For this review, use the dimensioned drawing (mm, ordinates from the lowest corner) and the shaded views. A direction names the side the tool comes from. Round coordinates to 2 decimals unless told otherwise and drop trailing zeros. Write each loop counter-clockwise with the first axis right and the second up, starting at its lowest first coordinate (ties: lowest second). Pieces come first, ordered by that corner, then holes. Notation, with made-up numbers: (1.25, 29.5) - (28.25, 29.5) arc R36 cw to (28.25, 65.5) - close; hole circle Ø5 at (-34.75, 20.25). An arc over 180 degrees is marked (long way). Return JSON: item names as keys, results as strings.
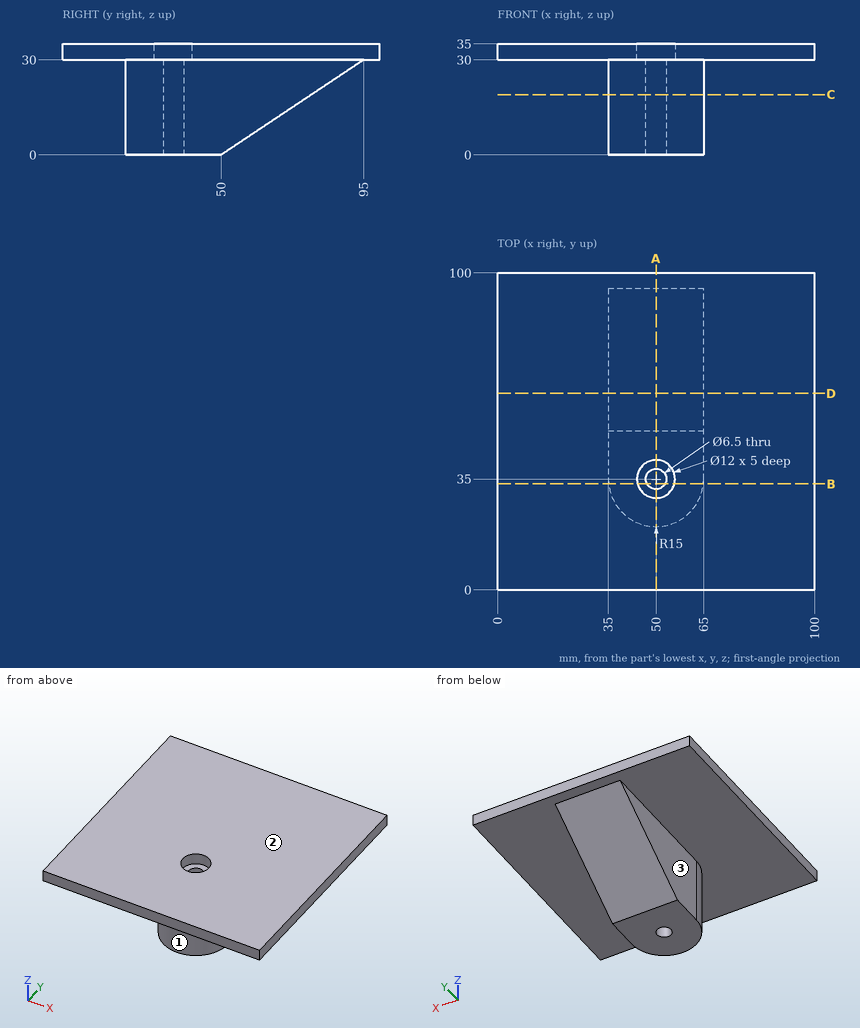
(1) Clearance check with flat-ended pins moving along their axes: pin 1 Ø5 at (x, z) = (34.5, 25.5) entering from -Y; pin 2 Ø5 at (y, z) = (82, 20) entering from +X; pin 3 Ø1 at (y, z) = (70.5, 22.5) entering from -X. State where each tip first meets the part, or that it passes through.
Filled in:
{"pin 1": "stops at y = 27.52", "pin 2": "stops at x = 65", "pin 3": "stops at x = 35"}
(2) Add section A-A (x = 50). Write out the cut boundary in (y, z).
Filled in:
{"outline": "(0, 30) - (20, 30) - (20, 0) - (31.75, 0) - (31.75, 30) - (29, 30) - (29, 35) - (0, 35) - close; (38.25, 0) - (50, 0) - (95, 30) - (100, 30) - (100, 35) - (41, 35) - (41, 30) - (38.25, 30) - close"}
(3) Add section C-C (z = 19). Write out the cut boundary in (x, y), plus the area to 3 significant figures.
Filled in:
{"outline": "(35, 35) arc R15 ccw to (65, 35) - (65, 78.5) - (35, 78.5) - close; hole circle Ø6.5 at (50, 35)", "area": "1,630 mm2"}
(4) Wall thickness on line 1 (Y direction, x = 50, z = 31.2); line 2 (X direction, y = 39.5, z = 9.5); line 3 (Z direction, x = 27, y = 89): over which ranges is each line inside the solid? List them lowest first.
Filled in:
{"line 1": "y = 0 to 29, 41 to 100", "line 2": "x = 35 to 65", "line 3": "z = 30 to 35"}
(5) Add section D-D (y = 62). Write out the cut boundary in (x, z), plus the area to 3 significant figures.
Filled in:
{"outline": "(0, 30) - (35, 30) - (35, 8) - (65, 8) - (65, 30) - (100, 30) - (100, 35) - (0, 35) - close", "area": "1,160 mm2"}
(6) Add section B-B (y = 33.5). Write out the cut boundary in (x, z), plus the area to 3 significant figures.
Filled in:
{"outline": "(0, 30) - (35.08, 30) - (35.08, 0) - (47.12, 0) - (47.12, 30) - (44.19, 30) - (44.19, 35) - (0, 35) - close; (52.88, 0) - (64.92, 0) - (64.92, 30) - (100, 30) - (100, 35) - (55.81, 35) - (55.81, 30) - (52.88, 30) - close", "area": "1,160 mm2"}
(7) For the marked faces 1, 2 and 3, list the 3-axis set-ups (+Z, -Z, +X, -X, +Y, -Y) from which the entire face can be reached by the end or side of a thin tool; tool diameter is ignored.
Filled in:
{"face 1": "-Z, -Y", "face 2": "+Z, +X, -X, +Y, -Y", "face 3": "-Z, -X, +Y, -Y"}
